```python
from build123d import *

# Parameters (mm, degrees)
F0_W     = 88.9
F0_H     = 50.8
F1_DEPTH = 10.16
F2_R     = 2.38125
F2_R_2   = 3.175
F3_DEPTH = 25.4
F4_W     = 66.04
F4_H     = 31.75
F5_DEPTH = 6.985
F6_W     = 58.42
F6_H     = 13.8684
F7_DEPTH = 1.27
F8_W     = 50.8
F8_H     = 11.43
F9_DEPTH = 25.4
F10_SIZE = 0.254


with BuildPart() as f1:
    # F0 (on Top) → F1 (new body)
    with BuildSketch(Plane.XY):
        with Locations((44.45, 25.4)):
            Rectangle(F0_W, F0_H)
    extrude(amount=F1_DEPTH)

    # F2 (on face) → F3 (cut)
    with BuildSketch(Plane.XY.offset(10.16)):
        with Locations((4.0132, 25.4)):
            Circle(F2_R)
        with Locations((82.804, 25.4)):
            Circle(F2_R_2)
    extrude(amount=-F3_DEPTH, mode=Mode.SUBTRACT)

    # F4 (on face) → F5 (cut)
    with BuildSketch(Plane(origin=(0, 0, 0), x_dir=(1, 0, 0), z_dir=(0, 0, -1))):
        with Locations((43.18, -25.4)):
            Rectangle(F4_W, F4_H)
    extrude(amount=-F5_DEPTH, mode=Mode.SUBTRACT)

    # F6 (on face) → F7 (cut)
    with BuildSketch(Plane(origin=(0, 0, 6.985), x_dir=(1, 0, 0), z_dir=(0, 0, -1))):
        with Locations((44.45, -25.4)):
            Rectangle(F6_W, F6_H)
    extrude(amount=-F7_DEPTH, mode=Mode.SUBTRACT)

    # F8 (on face) → F9 (cut)
    with BuildSketch(Plane(origin=(0, 0, 8.255), x_dir=(1, 0, 0), z_dir=(0, 0, -1))):
        with Locations((44.45, -25.4)):
            Rectangle(F8_W, F8_H)
    extrude(amount=-F9_DEPTH, mode=Mode.SUBTRACT)

    # F10
    f10_edges = [f1.edges().sort_by_distance(p)[0] for p in [
        (44.45, 31.115, 8.255),
        (69.85, 25.4, 8.255),
        (44.45, 19.685, 10.16),
        (19.05, 25.4, 8.255),
    ]]
    chamfer(f10_edges, length=F10_SIZE)


solid = f1.part
```
Here's how the part is built. I have some questions about the finished solid (model axes, mm). A direction names the side the tool comes from. Give positions to 0.01 mm unless a question says otherwise; leave off trailing zeros. Loops run counter-clockwise (first coordinate to the right, second up) from the corner with the lowest first, then second, coordinate; pieces in that order, holes last. Notation, with made-up numbers: (46, 24.25) -> (94, 24.25) arc R12 cw to (94, 45.25) -> close; hole circle Ø2 at (7.25, 15.5). An arc over 180 degrees is marked (long way). Use one line per item in the form item = value. Start each with the question number.
1) Imagine slicing it at B-B (y = 25.4). Please give me the cut outline in (x, z) (3 decimals).
2) For P1, Ø9.5, axis at x = 30, y = 31, coming from the -Z side (3 decimals); P2, Ø7, axis at x = 52.5, y = 28, coming from the -Z side (3 decimals); P3, Ø4, axis at x = 82.804, y = 25.4, coming from the -Z side, each with a flat end and sliding along its axis, tell me the tip position at first contact or that it passes through.
3) Thinking about a two-plate mould opening in X: for faces 4 (the face through (88.9, 25, 5)), 5 (the face through (43.8, 31.4, 10.16)), 6 (the face through (43, 18, 6.985)), 7 (the face through (2.26, 27.01, 5.15)), which applies, +X half, -X half, draft (parallel to the pull), parting line (faces both ways), or undercut?
4) Please list where these lines run through material, in increasing order: line 1 along Y through (x, z) = (26, 3.5) (3 decimals); line 2 along X through (y, z) = (19, 7.5); line 3 along Y through (x, z) = (68.5, 7.25).
5) Which directions (+Z, -Z, +X, -X, +Y, -Y) give clear straight access to the entire face, cutting with the end or side of a thin tool? Please do faces 1 (the face through (44, 19.685, 9)), 2 (the face through (44, 50.8, 5)), 3 (the face through (43, 9.525, 3)).
6) Imagine slicing it at A-A (z = 3.25). Count the separate pieces of the cut face and the enclosed holes in it, then the cut area to 3 significant figures.
7) Imagine slicing it at C-C (y = 35.5). Please give me the cut outline in (x, z) (3 decimals).
Check values:
q1.outline = (0, 0) -> (1.632, 0) -> (1.632, 10.16) -> (0, 10.16) -> close; (6.394, 0) -> (10.16, 0) -> (10.16, 6.985) -> (15.24, 6.985) -> (15.24, 8.255) -> (18.796, 8.255) -> (19.05, 8.509) -> (19.05, 10.16) -> (6.394, 10.16) -> close; (69.85, 8.509) -> (70.104, 8.255) -> (73.66, 8.255) -> (73.66, 6.985) -> (76.2, 6.985) -> (76.2, 0) -> (79.629, 0) -> (79.629, 10.16) -> (69.85, 10.16) -> close; (85.979, 0) -> (88.9, 0) -> (88.9, 10.16) -> (85.979, 10.16) -> close
q2.P1 = 6.985
q2.P2 = 8.255
q2.P3 = through
q3.face_4 = +X half
q3.face_5 = draft
q3.face_6 = undercut
q3.face_7 = undercut
q4.line_1 = 0 to 9.525, 41.275 to 50.8
q4.line_2 = 0 to 15.24, 73.66 to 88.9
q4.line_3 = 0 to 18.47, 32.33 to 50.8
q5.face_1 = +Z, -Z
q5.face_2 = +Z, -Z, +X, -X, +Y
q5.face_3 = -Z
q6.separate_pieces = 1
q6.enclosed_holes = 3
q6.area = 2,370 mm^2
q7.outline = (0, 0) -> (10.16, 0) -> (10.16, 6.985) -> (76.2, 6.985) -> (76.2, 0) -> (88.9, 0) -> (88.9, 10.16) -> (0, 10.16) -> close
